Could you check a few things on this model? Use its own coordinates, in mm. Give positions to 0.01 mm unless a question says otherwise; leave off trailing zeros. Loops run counter-clockwise (first coordinate to the right, second up) from the corner with the lowest first, then second, coordinate; pieces in that order, holes last. Notation, with made-up numbers: (-15.75, 70) - (17.25, 70) arc R6 cw to (17.25, 79) - close; hole circle Ø2 at (-35.75, 68). An arc over 180 degrees is marked (long way). Use CSV: the item, a comma, the result in double quotes.
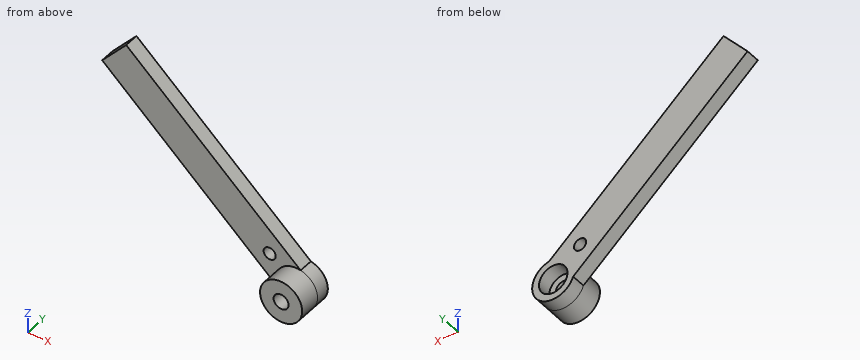
from build123d import *

# Parameters (mm, degrees)
EXTRUDE_START       = -4
EXTRUDE_1_OUTLINE_R = 4
EXTRUDE_1_DEPTH     = 4
EXTRUDE_START_2     = 6
SKETCH_2_R          = 5.9
SKETCH_2_R_2        = 2.1
EXTRUDE_2_DEPTH     = 6
SKETCH_3_R          = 1.7
CUT_EXTRUDE_1_DEPTH = 4


# Read off the part's stored shape, not the designer's step: 填料-伸長1
with BuildPart() as part:
    # 填料-伸長1 outline → 填料-伸長1 (new body)
    with BuildSketch(Plane(origin=(0, 20.156954032, 0), x_dir=(1, 0, 0), z_dir=(0, 1, 0)).offset(EXTRUDE_START)):
        with BuildLine():
            Line((-102.099122719, -450.012320429), (-53.224889363, -407.160140626))
            ThreePointArc((-53.224889363, -407.160140626), (-49.935495794, -397.483024153), (-59.959608209, -399.47898597))
            Line((-59.959608209, -399.47898597), (-108.833841565, -442.331165772))
            Line((-108.833841565, -442.331165772), (-102.099122719, -450.012320429))
        make_face()
        with Locations((-54.371772361, -401.372683552)):
            Circle(EXTRUDE_1_OUTLINE_R, mode=Mode.SUBTRACT)
    extrude(amount=EXTRUDE_1_DEPTH)

    # 草圖2 → 填料-伸長2 (add)
    with BuildSketch(Plane.XZ.offset(-16.156954032).offset(EXTRUDE_START_2)):
        with Locations(Location((-54.371772361, 401.372683552, 0), (0, 0, 198.721335886))):
            Circle(SKETCH_2_R)
        with Locations((-54.371772361, 401.372683552)):
            Circle(SKETCH_2_R_2, mode=Mode.SUBTRACT)
    extrude(amount=-EXTRUDE_2_DEPTH)

    # 草圖3 → 除料-伸長1 (cut)
    with BuildSketch(Plane.XZ.offset(-16.156954032)):
        with Locations((-61.890885185, 407.965326598)):
            Circle(SKETCH_3_R)
    extrude(amount=-CUT_EXTRUDE_1_DEPTH, mode=Mode.SUBTRACT)


solid = part.part
1) Suppose I cut it at B-B (x = -66). Please give me the cut outline in (y, z).
Answer below:
outline,"(16.16, 404.78) - (20.16, 404.78) - (20.16, 418.36) - (16.16, 418.36) - close"
2) Suppose I cut it at D-D (z = 445). Please give me the cut outline in (x, y).
Answer below:
outline,"(-106.49, 16.16) - (-96.38, 16.16) - (-96.38, 20.16) - (-106.49, 20.16) - close"
3) Suppose I cut it at C-C (y = 18.75). Please give me the cut outline in (x, z).
Answer below:
outline,"(-108.83, 442.33) - (-59.96, 399.48) arc R5.9 ccw (long way) to (-53.22, 407.16) - (-102.1, 450.01) - close; hole circle Ø3.4 at (-61.89, 407.97); hole circle Ø8 at (-54.37, 401.37)"
4) Suppose I cut it at A-A (y = 15.5). Please give me the cut outline in (x, z), plus the area to 3 significant figures.
Answer below:
outline,"circle Ø11.8 at (-54.37, 401.37); hole circle Ø4.2 at (-54.37, 401.37)"
area,"95.5 mm2"
5) I need wall thicknesses on line 1 along X through (y, z) = (11, 400.5); line 2 along Y through (x, z) = (-59, 411.5); line 3 along X through (y, z) = (19.75, 443). Which ranges of each line are inside material? Lowest first, please.
Answer below:
line 1,"x = -60.21 to -56.28, -52.46 to -48.54"
line 2,"y = 16.16 to 20.16"
line 3,"x = -108.25 to -94.1"
6) I'm going to push flat-ended pins straight in: P1, Ø10.5, axis at x = -54.37, z = 401.37, coming from the -Y side; P2, Ø5.5, axis at x = -61.89, z = 407.97, coming from the -Y side; P3, Ø1.5, axis at x = -82, y = 16.5, coming from the +Z side; P4, Ø3, axis at y = 14.5, z = 411, coming from the +X side. Where does each tip first touch, or does it pass through?
Answer below:
P1,"stops at y = 10.16"
P2,"stops at y = 16.16"
P3,"stops at z = 433.05"
P4,"passes through"
